Autodesk Inventor part; units mm, degrees
ref_plane "YZ Plane" through (0, 0, 0) normal (1, 0, 0) x (0, 1, 0)
ref_plane "XZ Plane" through (0, 0, 0) normal (0, 1, 0) x (-1, 0, 0)
ref_plane "XY Plane" through (0, 0, 0) normal (0, 0, 1) x (1, 0, 0)
sketch "Sketch1" plane through (0, 0, 0) normal (1, 0, 0) x (0, 1, 0)
  line L0 (10.57, 0) -> (0, 0)
  line L1 (0, 0) -> (0, -17.74)
  line L2 (0, -17.74) -> (10.57, -17.74)
  line L3 (10.57, -17.74) -> (10.57, 0)
  circle A0 centre (5.285, 2.5) radius 2.5
  circle A1 centre (5.285, 2.5) radius 1.5
  line L4 (10.57, -8.87) -> (0, -8.87) construction
  circle A2 centre (5.285, -20.24) radius 2.5
  circle A3 centre (5.285, -20.24) radius 1.5
  line L5 (7.785, 2.5) -> (7.785, 0)
  line L6 (2.785, 2.5) -> (2.785, 0)
  line L7 (7.785, -20.24) -> (7.785, -17.74)
  line L8 (2.785, -20.24) -> (2.785, -17.74)
  dimension "d0" = 17.74
  dimension "d1" = 10.57
  dimension "d2" = 5.285
  dimension "d3" = 5
  dimension "d11" = 3
extrude "Extrusion1" add sketch "Sketch1" against normal blind 1.57
properties part number "VL53L1X board"
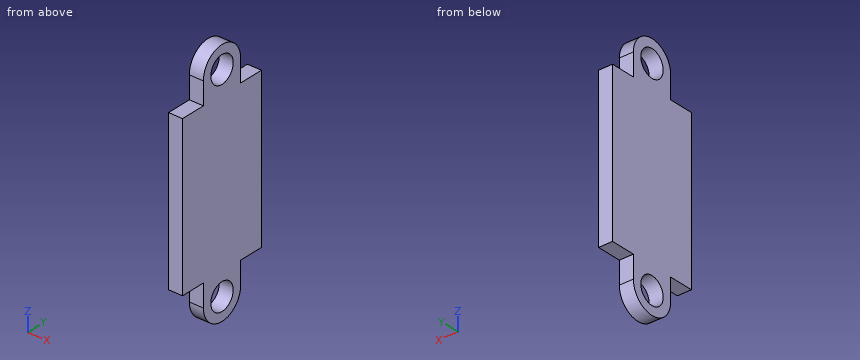
CAD build for the part. Positions are in the model's coordinates, mm. Give positions to 0.01 mm unless a question says otherwise; leave off trailing zeros. Loops run counter-clockwise (first coordinate to the right, second up) from the corner with the lowest first, then second, coordinate; pieces in that order, holes last. Notation, with made-up numbers: (76.25, 87.25) - (103.25, 87.25) arc R25 cw to (103.25, 114.25) - close; hole circle Ø5 at (-15.75, 66.25). An arc over 180 degrees is marked (long way). Put each result on its own line as item: value.
Q1. Slice it at C-C (z = -19). Give the cut face in (x, y) (3 decimals).
Filled in:
outline: (-1.57, 2.785) - (0, 2.785) - (0, 4.441) - (-1.57, 4.441) - close; (-1.57, 6.129) - (0, 6.129) - (0, 7.785) - (-1.57, 7.785) - close
Q2. Flat gauge pins, fed straight in: pin 1 (0.8 mm diameter, centred on x = -0.5, z = 1, fed in from -Y) (3 decimals); pin 2 (0.8 mm diameter, centred on x = -0.5, y = 1.5, fed in from +Z); pin 3 (0.8 mm diameter, centred on x = -1, y = 9, fed in from -Z). Where does each tip first touch, or does it go through?
Filled in:
pin 1: stops at y = 2.785
pin 2: stops at z = 0
pin 3: stops at z = -17.74
Q3. Probe line 1 along Z through (x, y) = (-0.4, 5.25); line 2 along Z through (x, y) = (-1.3, 6); line 3 along Z through (x, y) = (-0.7, 1.5). List the from-to ranges inside material, lowest first.
Filled in:
line 1: z = -22.74 to -21.74, -18.74 to 1, 4 to 5
line 2: z = -22.64 to -21.56, -18.92 to 1.18, 3.82 to 4.9
line 3: z = -17.74 to 0
Q4. Slice it at B-B (y = 5.5). Give the cut face in (x, z), plus the area to 3 significant figures.
Filled in:
outline: (-1.57, -22.73) - (0, -22.73) - (0, -21.72) - (-1.57, -21.72) - close; (-1.57, -18.76) - (0, -18.76) - (0, 1.02) - (-1.57, 1.02) - close; (-1.57, 3.98) - (0, 3.98) - (0, 4.99) - (-1.57, 4.99) - close
area: 34.2 mm²
Q5. Slice it at A-A (x = -0.35). Give the cut face in (y, z) (3 decimals).
Filled in:
outline: (0, -17.74) - (2.785, -17.74) - (2.785, -20.24) arc R2.5 ccw to (7.785, -20.24) - (7.785, -17.74) - (10.57, -17.74) - (10.57, 0) - (7.785, 0) - (7.785, 2.5) arc R2.5 ccw to (2.785, 2.5) - (2.785, 0) - (0, 0) - close; hole circle Ø3 at (5.285, -20.24); hole circle Ø3 at (5.285, 2.5)
Q6. Slice it at D-D (y = 2.5). Give the cut face in (x, z).
Filled in:
outline: (-1.57, -17.74) - (0, -17.74) - (0, 0) - (-1.57, 0) - close
